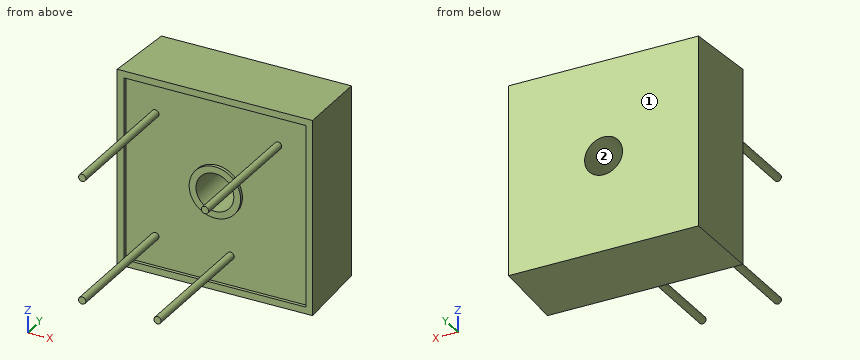
from build123d import *

# Parameters (mm, degrees)
SKETCH1_W           = 28.8
SKETCH1_H           = 28.8
BOSS_EXTRUDE1_DEPTH = 11.23
BOSS_EXTRUDE1_TAPER = 2
SKETCH2_W           = 26.8
SKETCH2_H           = 26.8
SKETCH2_R           = 3.795
CUT_EXTRUDE1_DEPTH  = 0.5
SKETCH3_R           = 2.795
CUT_EXTRUDE2_DEPTH  = 24.255814499
BOSS_EXTRUDE2_START = -10.73
SKETCH4_R           = 0.535
BOSS_EXTRUDE2_DEPTH = 30.5


with BuildPart() as part:
    # Sketch1 → Boss-Extrude1 (new body)
    with BuildSketch(Plane(origin=(0, 0, 0), x_dir=(1, 0, 0), z_dir=(0, 1, 0))):
        Rectangle(SKETCH1_W, SKETCH1_H)
    extrude(amount=BOSS_EXTRUDE1_DEPTH, taper=BOSS_EXTRUDE1_TAPER)

    # Sketch2 → Cut-Extrude1 (cut)
    with BuildSketch(Plane.XZ):
        Rectangle(SKETCH2_W, SKETCH2_H)
        with Locations(Location((0, 0, 0), (0, 0, 270))):
            Circle(SKETCH2_R, mode=Mode.SUBTRACT)
    extrude(amount=-CUT_EXTRUDE1_DEPTH, mode=Mode.SUBTRACT)

    # Sketch3 → Cut-Extrude2 (cut, through all)
    with BuildSketch(Plane.XZ):
        with Locations(Location((0, 0, 0), (0, 0, 270))):
            Circle(SKETCH3_R)
    extrude(amount=-CUT_EXTRUDE2_DEPTH, mode=Mode.SUBTRACT)

    # Sketch4 → Boss-Extrude2 (add)
    with BuildSketch(Plane.XZ.offset(-0.5).offset(BOSS_EXTRUDE2_START)):
        with Locations(Location((-9.05, 9.05, 0), (0, 0, 90))):
            Circle(SKETCH4_R)
        with Locations(Location((9.05, 9.05, 0), (0, 0, 90))):
            Circle(SKETCH4_R)
        with Locations(Location((-9.05, -9.05, 0), (0, 0, 90))):
            Circle(SKETCH4_R)
        with Locations(Location((2.05, -9.05, 0), (0, 0, 90))):
            Circle(SKETCH4_R)
    extrude(amount=BOSS_EXTRUDE2_DEPTH)


solid = part.part
Geometry: final body of the model. Coordinates: model frame, mm. Face numbers are marked on the shaded views. Round coordinates to 2 decimals unless told otherwise and drop trailing zeros. Order: outer loops, then holes, each group sorted by start corner. A loop starts at its lowest first (then second) coordinate and runs counter-clockwise, first axis right, second up. Notation, with made-up numbers: (-35, 11) -> (17, 11) arc R30 ccw to (17, 34) -> close; hole circle Ø10 at (60.25, 37). An arc over 180 degrees is marked (long way). Put each result on its own line as item: value. Start each with the question number.
Q1. Pull-direction query (Z, two-part tool) for the marked faces 1 and 2; classes: +Z half, -Z half, draft (parallel to the pull), parting line (faces both ways), or undercut.
Q2. Section A-A on y = -6.5. Return the cut outline in (x, z) (3 decimals).
Q3. First-contact query: pin 1 (9 mm diameter, centred on x = 0, z = 0, fed in from -Y); pin 2 (1.5 mm diameter, centred on x = 2.5, z = 8.5, fed in from -Y); pin 3 (8 mm diameter, centred on x = -6, y = -9.5, fed in from -Z) (3 decimals). Flat tips, straight axial feed; report the tip coordinate or a pass-through.
Q4. Line query: probe 1 along Y at (x, z) = (-3, 11); probe 2 along X at (y, z) = (6.5, 0) (3 decimals); probe 3 along Z at (x, y) = (9, -13.5). Output: solid intervals per line, ascending.
Ans:
1. face 1: draft
1. face 2: undercut
2. outline: circle Ø1.07 at (-9.05, -9.05); circle Ø1.07 at (-9.05, 9.05); circle Ø1.07 at (2.05, -9.05); circle Ø1.07 at (9.05, 9.05)
3. pin 1: stops at y = 0
3. pin 2: stops at y = 0.5
3. pin 3: stops at z = -9.585
4. probe 1: y = 0.5 to 11.23
4. probe 2: x = -14.173 to -2.795, 2.795 to 14.173
4. probe 3: z = 8.52 to 9.58
